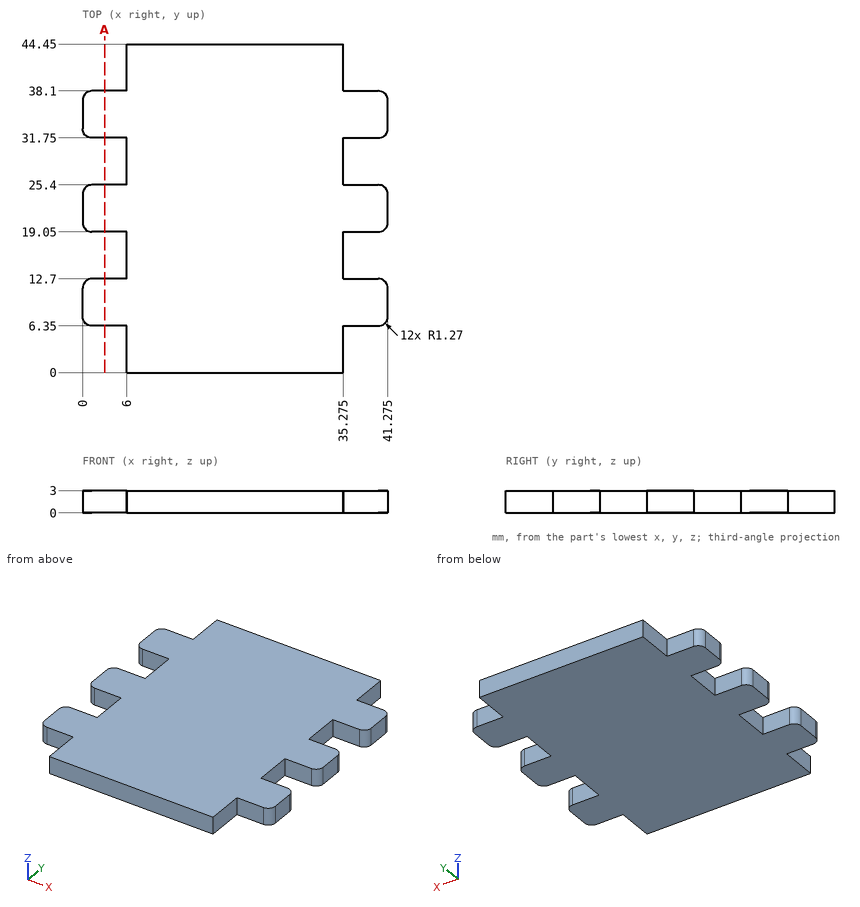
Geometry check sheet. Reference: drawing and pictorial views, mm from the part's lowest x, y, z. Coordinates: 2 decimals unless noted, no trailing zeros. Order: outer loops, then holes, each group sorted by start corner. A loop starts at its lowest first (then second) coordinate and runs counter-clockwise, first axis right, second up. Notation, with made-up numbers: M 24.25,52.25 L 58.25,52.25 A26 ccw 58.25,66.25 Z; hole C 6.25,21 d4. An arc over 180 degrees is marked long. Return JSON: item names as keys, results as strings.
1) Gauge pin test, flat ends, axial feed: pin 1 (0.9 mm diameter, centred on y = 2, z = 2, fed in from +X) (3 decimals); pin 2 (0.9 mm diameter, centred on x = 38, z = 1.5, fed in from -Y); pin 3 (0.9 mm diameter, centred on x = 38, z = 1.5, fed in from +Y). Record the tip position at first contact, or that the pin passes through.
Answer list:
{"pin 1": "x = 35.275", "pin 2": "y = 6.35", "pin 3": "y = 38.1"}
2) Thickness scan on L1, parallel to Y at x = 5, z = 2.35; L2, parallel to X at y = 11.5, z = 2.85; L3, parallel to X at y = 19, z = 2.6 (3 decimals). Record the ranges inside material, lowest first. Write a range as [from, to].
Answer list:
{"L1": "[6.35, 12.7], [19.05, 25.4], [31.75, 38.1]", "L2": "[0, 41.27]", "L3": "[6, 35.275]"}
3) Cross-section at A-A, the plane x = 3. Record the boundary of the cut face in (y, z).
Answer list:
{"outline": "M 6.35,0 L 12.7,0 L 12.7,3 L 6.35,3 Z; M 19.05,0 L 25.4,0 L 25.4,3 L 19.05,3 Z; M 31.75,0 L 38.1,0 L 38.1,3 L 31.75,3 Z"}
